Design review of the part built by this model. Coordinates are the model's own, in mm. A direction names the side the tool comes from. Give positions to 0.01 mm unless a question says otherwise; leave off trailing zeros. Write each loop counter-clockwise with the first axis right and the second up, starting at its lowest first coordinate (ties: lowest second). Pieces come first, ordered by that corner, then holes. Notation, with made-up numbers: M 57.25,-13 L 93.25,-13 A15 ccw 93.25,-2 Z; hole C -19,-20 d9. An arc over 180 degrees is marked long. Answer in a Markdown table with one row per item.
```python
from build123d import *

# Parameters (mm, degrees)
SKETCH1_W           = 32
SKETCH1_H           = 32
SKETCH1_R           = 1
BOSS_EXTRUDE1_DEPTH = 1.2
SKETCH2_R           = 5
BOSS_EXTRUDE2_DEPTH = 14
SKETCH3_W           = 10
SKETCH3_H           = 6
BOSS_EXTRUDE3_DEPTH = 8


with BuildPart() as part:
    # Sketch1 → Boss-Extrude1 (new body)
    with BuildSketch(Plane(origin=(0, 0, 0), x_dir=(1, 0, 0), z_dir=(0, 1, 0))):
        Rectangle(SKETCH1_W, SKETCH1_H)
        with Locations(Location((-14, 14, 0), (0, 0, 270))):
            Circle(SKETCH1_R, mode=Mode.SUBTRACT)
        with Locations(Location((14, 14, 0), (0, 0, 270))):
            Circle(SKETCH1_R, mode=Mode.SUBTRACT)
        with Locations(Location((14, -14, 0), (0, 0, 270))):
            Circle(SKETCH1_R, mode=Mode.SUBTRACT)
        with Locations(Location((-14, -14, 0), (0, 0, 270))):
            Circle(SKETCH1_R, mode=Mode.SUBTRACT)
    extrude(amount=BOSS_EXTRUDE1_DEPTH)

    # Sketch2 → Boss-Extrude2 (add)
    with BuildSketch(Plane(origin=(0, 1.2, 0), x_dir=(1, 0, 0), z_dir=(0, 1, 0))):
        with Locations(Location((0, 0, 0), (0, 0, 270))):
            Circle(SKETCH2_R)
    extrude(amount=BOSS_EXTRUDE2_DEPTH)

    # Sketch3 → Boss-Extrude3 (add)
    with BuildSketch(Plane.XZ):
        with Locations((4, 11)):
            Rectangle(SKETCH3_W, SKETCH3_H)
    extrude(amount=BOSS_EXTRUDE3_DEPTH)


solid = part.part
```
1) Add section D-D (y = 11). Write out the cut boundary in (x, z), and give its area (3 significant figures).
Geometry says:
| item | result |
|---|---|
| outline | C 0,0 d10 |
| area | 78.5 mm^2 |
2) The part is to be moulded in two halves that separate along Z. For faces 1 (the face through (0, 1, 16)), 2 (the face through (-4, 1.2, -4)), 3 (the face through (-15, 1, -14)), 4 (the face through (4, -4, 8)), say which applies: released by +Z, released by -Z, zero draft, split by the parting line, or undercut.
Geometry says:
| item | result |
|---|---|
| face 1 | released by +Z |
| face 2 | zero draft |
| face 3 | undercut |
| face 4 | released by -Z |
3) For faces 5 (the face through (-4.88, 8.1, -1.08)), 6 (the face through (9, -4, 11)), 7 (the face through (4, -4, 14)), 8 (the face through (-1, -4, 11)), list the 3-axis set-ups (+Z, -Z, +X, -X, +Y, -Y) from which the entire face can be reached by the end or side of a thin tool; tool diameter is ignored.
Geometry says:
| item | result |
|---|---|
| face 5 | +Y |
| face 6 | +Z, -Z, +X, -Y |
| face 7 | +Z, +X, -X, -Y |
| face 8 | +Z, -Z, -X, -Y |
4) Add section B-B (z = 3). Write out the cut boundary in (x, y).
Geometry says:
| item | result |
|---|---|
| outline | M -16,0 L 16,0 L 16,1.2 L 4,1.2 L 4,15.2 L -4,15.2 L -4,1.2 L -16,1.2 Z |
5) Insertion check: P1, Ø1.5, axis at x = -10, z = -11, coming from the +Y side; P2, Ø1.8, axis at y = -3, z = 12, coming from the +X side; P3, Ø9.5, axis at x = -2.5, z = -5, coming from the -Y side; P4, Ø6.5, axis at y = -2, z = 11, coming from the -X side. Each pin has a flat end and moves straight along its axis. Give the tip position at first contact, or say it passes through.
Geometry says:
| item | result |
|---|---|
| P1 | y = 1.2 |
| P2 | x = 9 |
| P3 | y = 0 |
| P4 | x = -16 |
6) To check wall thickness, follow probe 1 along X at (y, z) = (0.7, -14); probe 2 along Y at (x, z) = (5, 8.5); probe 3 along Y at (x, z) = (4, -7). State the ranges of each line that lie inside material, in increasing order. Write a range as [from, to].
Geometry says:
| item | result |
|---|---|
| probe 1 | [-16, -15], [-13, 13], [15, 16] |
| probe 2 | [-8, 1.2] |
| probe 3 | [0, 1.2] |
7) Add section A-A (x = -14). Write out the cut boundary in (y, z).
Geometry says:
| item | result |
|---|---|
| outline | M 0,-16 L 1.2,-16 L 1.2,-15 L 0,-15 Z; M 0,-13 L 1.2,-13 L 1.2,13 L 0,13 Z; M 0,15 L 1.2,15 L 1.2,16 L 0,16 Z |
8) Add section C-C (x = 0). Write out the cut boundary in (y, z), and give its area (3 significant figures).
Geometry says:
| item | result |
|---|---|
| outline | M -8,8 L 0,8 L 0,-16 L 1.2,-16 L 1.2,-5 L 15.2,-5 L 15.2,5 L 1.2,5 L 1.2,16 L 0,16 L 0,14 L -8,14 Z |
| area | 226 mm^2 |
